from build123d import *

# Parameters (mm, degrees)
SKETCH1_R           = 82.5246
BOSS_EXTRUDE1_DEPTH = 38.1
SKETCH2_R           = 57.15
CUT_EXTRUDE1_DEPTH  = 38.1
SKETCH3_R           = 3.5687
CUT_EXTRUDE3_DEPTH  = 123.769007532
SKETCH4_R           = 5.5626
CUT_EXTRUDE4_DEPTH  = 9.652
CHAMFER1_SIZE       = 1.524


with BuildPart() as part:
    # Sketch1 → Boss-Extrude1 (new body)
    with BuildSketch(Plane.YZ):
        with Locations(Location((0, 0, 0), (0, 0, 270))):
            Circle(SKETCH1_R)
    extrude(amount=BOSS_EXTRUDE1_DEPTH)

    # Sketch2 → Cut-Extrude1 (cut)
    with BuildSketch(Plane.YZ):
        with Locations(Location((0, 0, 0), (0, 0, 270))):
            Circle(SKETCH2_R)
    extrude(amount=CUT_EXTRUDE1_DEPTH, mode=Mode.SUBTRACT)

    # Sketch3 → Cut-Extrude3 (cut, through all)
    with BuildSketch(Plane.YZ):
        with Locations(Location((0, 73.025, 0), (0, 0, 270))):
            Circle(SKETCH3_R)
        with Locations(Location((-63.241505111, -36.5125, 0), (0, 0, 270))):
            Circle(SKETCH3_R)
        with Locations(Location((63.241505111, -36.5125, 0), (0, 0, 270))):
            Circle(SKETCH3_R)
    extrude(amount=CUT_EXTRUDE3_DEPTH, mode=Mode.SUBTRACT)

    # Sketch4 → Cut-Extrude4 (cut)
    with BuildSketch(Plane.YZ):
        with Locations(Location((0, 73.025, 0), (0, 0, 270))):
            Circle(SKETCH4_R)
        with Locations(Location((-63.241505111, -36.5125, 0), (0, 0, 270))):
            Circle(SKETCH4_R)
        with Locations(Location((63.241505111, -36.5125, 0), (0, 0, 270))):
            Circle(SKETCH4_R)
    extrude(amount=CUT_EXTRUDE4_DEPTH, mode=Mode.SUBTRACT)

    # Chamfer1
    chamfer1_edges = [part.edges().sort_by_distance(p)[0] for p in [
        (0, 0, 82.5246),
        (38.1, 0, 82.5246),
    ]]
    chamfer(chamfer1_edges, length=CHAMFER1_SIZE)


solid = part.part
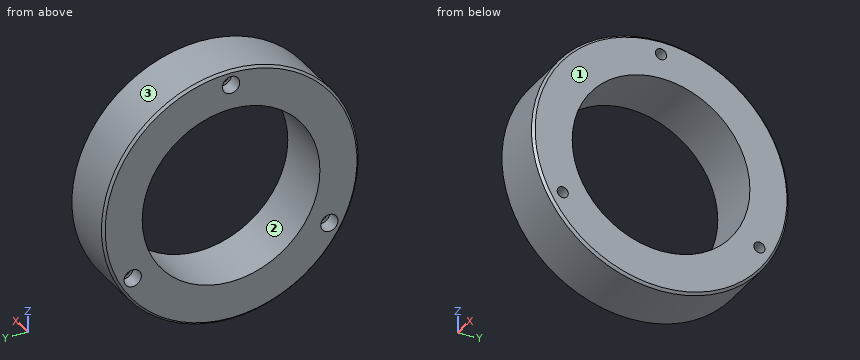
Can you work these out from the model? Positions are in its coordinate system, mm. Face numbers are marked on the shaded views. Coordinates: 2 decimals unless noted, no trailing zeros. Write each loop counter-clockwise with the first axis right and the second up, starting at its lowest first coordinate (ties: lowest second). Pieces come first, ordered by that corner, then holes. Notation, with made-up numbers: (-19.75, 23.25) -> (32.25, 23.25) arc R8 ccw to (32.25, 33.25) -> close; hole circle Ø9 at (53, 58). An arc over 180 degrees is marked (long way). Write each question's results on one line, items separated by ' | '. Start each with the question number.
Q1. Imagine slicing it at B-B (y = 0). Write out the boundary of the cut face in (x, z).
Q2. If I drill on probe 1 along Y at (x, z) = (20.5, 0); probe 2 along Z at (x, y) = (4, -28.5); probe 3 along Z at (x, y) = (34.5, -62), over which ranges is the centre line in solid material (lowest first)?
Q3. Imagine slicing it at C-C (x = 26). State how many separate pieces and enclosed holes the cut face has, then the cut area to 3 significant figures.
Q4. Imagine slicing it at A-A (z = 0). Write out the boundary of the cut face in (x, y).
Q5. I'm going to push flat-ended pins straight in: pin 1 (6 mm diameter, centred on x = 4.5, z = -21, fed in from -Y); pin 2 (1.5 mm diameter, centred on x = 22, z = -29.5, fed in from +Y); pin 3 (8 mm diameter, centred on y = -63.24, z = -36.51, fed in from +X); pin 4 (10 mm diameter, centred on y = 0, z = 73.025, fed in from -X). Where does each tip first touch, or does it pass through?
Q6. We'd pull the mould along Z, two halves only. Please class the marked faces 1, 2 and 3: +Z half, -Z half, draft (parallel to the pull), parting line (faces both ways), or undercut.
Taken from the geometry:
1) outline: (0, -81) -> (1.52, -82.52) -> (36.58, -82.52) -> (38.1, -81) -> (38.1, -57.15) -> (0, -57.15) -> close; (0, 57.15) -> (38.1, 57.15) -> (38.1, 69.46) -> (9.65, 69.46) -> (9.65, 67.46) -> (0, 67.46) -> close; (0, 78.59) -> (9.65, 78.59) -> (9.65, 76.59) -> (38.1, 76.59) -> (38.1, 81) -> (36.58, 82.52) -> (1.52, 82.52) -> (0, 81) -> close
2) probe 1: y = -82.52 to -57.15, 57.15 to 82.52 | probe 2: z = -77.45 to -49.54, 49.54 to 77.45 | probe 3: z = -54.46 to -39.86, -33.17 to 54.46
3) separate pieces: 1 | enclosed holes: 4 | area: 11,000 mm^2
4) outline: (0, -81) -> (1.52, -82.52) -> (36.58, -82.52) -> (38.1, -81) -> (38.1, -57.15) -> (0, -57.15) -> close; (0, 57.15) -> (38.1, 57.15) -> (38.1, 81) -> (36.58, 82.52) -> (1.52, 82.52) -> (0, 81) -> close
5) pin 1: stops at y = -80.54 | pin 2: stops at y = 77.35 | pin 3: stops at x = 38.1 | pin 4: stops at x = 9.65
6) face 1: draft | face 2: undercut | face 3: parting line
